Could you check a few things on this model? Use its own coordinates, in mm. A direction names the side the tool comes from. Give positions to 0.01 mm unless a question says otherwise; leave off trailing zeros. Write each loop counter-clockwise with the first axis right and the second up, starting at its lowest first coordinate (ties: lowest second). Pieces come first, ordered by that corner, then holes. Notation, with made-up numbers: (-29, -24.75) -> (11, -24.75) arc R19 cw to (11, 9.25) -> close; hole circle Ø11 at (-6.75, 39.25). An arc over 180 degrees is marked (long way). Write item = value, one per line. Start each with the question number.
```python
from build123d import *

# Parameters (mm, degrees)
CROQUIS1_R              = 0.5
SALIENTE_EXTRUIR1_DEPTH = 3
MATRIZC1_COUNT          = 4
CROQUIS2_R              = 5
CROQUIS2_R_2            = 3
SALIENTE_EXTRUIR2_DEPTH = 8.5
CHAFL_N1_SIZE           = 1
CHAFL_N1_SIZE2          = 0.577350269
REDONDEO1_R             = 1
CUT_EXTRUDE1_DEPTH      = 10


with BuildPart() as part:
    # Croquis1 → Saliente-Extruir1 (new body)
    with BuildSketch(Plane(origin=(0, 0, 0), x_dir=(1, 0, 0), z_dir=(0, 1, 0))):
        with BuildLine():
            Line((-4, 0), (-4, 6.574293681))
            ThreePointArc((-4, 6.574293681), (-3.974394349, 6.996885575), (-3.897952052, 7.413294188))
            Line((-3.897952052, 7.413294188), (-1.698976026, 16.319147094))
            ThreePointArc((-1.698976026, 16.319147094), (0, 17.649646841), (1.698976026, 16.319147094))
            Line((1.698976026, 16.319147094), (3.897952052, 7.413294188))
            ThreePointArc((3.897952052, 7.413294188), (3.974394349, 6.996885575), (4, 6.574293681))
            Line((4, 6.574293681), (4, 0))
            Line((4, 0), (1.25, 0))
            ThreePointArc((1.25, 0), (0, 1.25), (-1.25, 0))
            Line((-1.25, 0), (-4, 0))
        make_face()
        with Locations(Location((0, 15.899646841, 0), (0, 0, 270))):
            Circle(CROQUIS1_R, mode=Mode.SUBTRACT)
        with Locations(Location((0, 12.899646841, 0), (0, 0, 270))):
            Circle(CROQUIS1_R, mode=Mode.SUBTRACT)
        with Locations(Location((0, 9.899646841, 0), (0, 0, 270))):
            Circle(CROQUIS1_R, mode=Mode.SUBTRACT)
        with Locations(Location((0, 6.899646841, 0), (0, 0, 270))):
            Circle(CROQUIS1_R, mode=Mode.SUBTRACT)
    saliente_extruir1 = extrude(amount=SALIENTE_EXTRUIR1_DEPTH)

    # MatrizC1: Saliente-Extruir1 ×4 about axis
    matrizc1_axis = Axis((0, 0, 0), (0, 1, 0))
    for i in range(1, MATRIZC1_COUNT):
        add(saliente_extruir1.rotate(matrizc1_axis, i * 360 / MATRIZC1_COUNT))

    # Croquis2 → Saliente-Extruir2 (add)
    with BuildSketch(Plane(origin=(0, 3, 0), x_dir=(1, 0, 0), z_dir=(0, 1, 0))):
        with Locations(Location((0, 0, 0), (0, 0, 270))):
            Circle(CROQUIS2_R)
        with Locations(Location((0, 0, 0), (0, 0, 270))):
            Circle(CROQUIS2_R_2, mode=Mode.SUBTRACT)
    extrude(amount=SALIENTE_EXTRUIR2_DEPTH)

    # Chaflán1
    chafl_n1_edges = [part.edges().sort_by_distance(p)[0] for p in [
        (0, 11.5, -5),
    ]]
    chafl_n1_side = [part.faces().sort_by_distance(p)[0] for p in [
        (0, 7.25, -5),
    ]]
    chamfer(chafl_n1_edges, length=CHAFL_N1_SIZE, length2=CHAFL_N1_SIZE2, reference=chafl_n1_side[0])

    # Redondeo1
    redondeo1_edges = [part.edges().sort_by_distance(p)[0] for p in [
        (-4, 1.5, -4),
        (4, 1.5, -4),
        (4, 1.5, 4),
        (-4, 1.5, 4),
    ]]
    fillet(redondeo1_edges, radius=REDONDEO1_R)

    # Sketch1 → Cut-Extrude1 (cut)
    with BuildSketch(Plane.XZ):
        Polygon((4, 5), (-4, 5), (-4, 20.808082072), (5.438258964, 20.808082072), (5.438258964, 5), align=None)
        Polygon((5.438258964, -5), (4, -5), (-4, -5), (-4, -20.808082072), (5.438258964, -20.808082072), align=None)
    extrude(amount=-CUT_EXTRUDE1_DEPTH, mode=Mode.SUBTRACT)


solid = part.part
```
(1) Imagine slicing it at B-B (y = 4.75). Please give me the cut outline in (x, z).
(2) We'd pull the mould along Z, two halves only. Please class faces 1 (the cylindrical face through (4.285, 1.521, -4.301)), 2 (the flat face through (-11.804, 1.479, 2.814)), 3 (the cylindrical face through (-15.438, 1.479, 0.192)): released by +Z, released by -Z, zero draft, split by the parting line, or undercut.
(3) On a 3-axis mill with a long thin cutter (end or side, diameter ignored), from which of +Z, -Z, +X, -X, +Y, -Y can I reach the whole of each face in a straight line? I mean faces 4 (the flat face through (-3, 11.5, 1)), 5 (the cylindrical face through (0.9, 7.19, 2.86)), 6 (the flat face through (11.804, 1.479, -2.814)), 7 (the flat face through (-6, 1, 4)), 8 (the flat face through (6, 1, 4)). Say none if no direction works.
(4) Imagine slicing it at D-D (x = 7). Please give me the cut outline in (y, z), then the cut area to 3 significant figures.
(5) Imagine slicing it at A-A (y = 1.5). State how many separate pieces and enclosed holes the cut face has, then the cut area to 3 significant figures.
(6) If I drill on line 1 along Z through (x, y) = (0, 1.75); line 2 along Y through (x, z) = (-2, -1.5); line 3 along X through (y, z) = (6.25, -1), over which ranges is the centre line in solid material (lowest first)? Write a range as from..to.
(7) I'm going to push flat-ended pins straight in: pin 1 (3 mm diameter, centred on y = 6.5, z = 3.5, fed in from -X); pin 2 (4 mm diameter, centred on y = 8, z = 2, fed in from +X); pin 3 (3 mm diameter, centred on x = 12, z = 1, fed in from +Y). Where does each tip first touch, or does it pass through?
Answers below:
q1.outline = circle Ø10 at (0, 0); hole circle Ø6 at (0, 0)
q2.face_1 = released by -Z
q2.face_2 = released by +Z
q2.face_3 = undercut
q3.face_4 = +Z, -Z, +X, -X, +Y
q3.face_5 = +Y
q3.face_6 = -Z, +X, +Y, -Y
q3.face_7 = +Z, -X, +Y, -Y
q3.face_8 = +Z, +X, +Y, -Y
q4.outline = (0, -3.97) -> (3, -3.97) -> (3, -0.49) -> (0, -0.49) -> close; (0, 0.49) -> (3, 0.49) -> (3, 3.97) -> (0, 3.97) -> close
q4.area = 20.9 mm^2
q5.separate_pieces = 1
q5.enclosed_holes = 9
q5.area = 231 mm^2
q6.line_1 = -5..-1.25, 1.25..5
q6.line_2 = 0..3
q6.line_3 = -4.9..-2.83, 2.83..4.9
q7.pin_1 = -4.58
q7.pin_2 = 5
q7.pin_3 = 3
